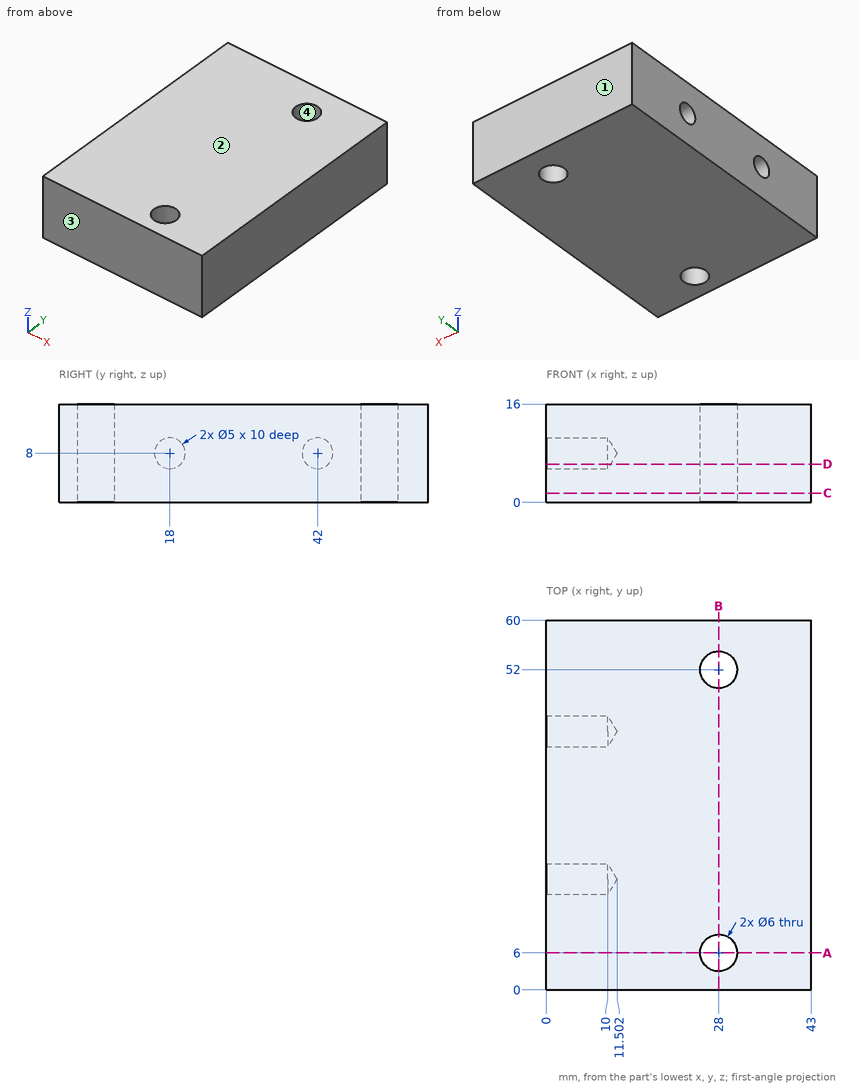
The drawing under review shows one solid part. Ordinate dimensions are in mm from its lowest x, y, z. Round coordinates to 2 decimals unless told otherwise and drop trailing zeros. Loops run counter-clockwise (first coordinate to the right, second up) from the corner with the lowest first, then second, coordinate; pieces in that order, holes last. Notation, with made-up numbers: M 27,-12.5 L 82,-12.5 A32 ccw 82,26.5 Z; hole C 83,82 d11. An arc over 180 degrees is marked long. Answer as CSV lines item,"result". Start each with the question number.
Item 1: Consider section A-A (y = 6). Write out the cut boundary in (x, z), then the cut area to 3 significant figures.
Item 2: Consider section D-D (z = 6.25). State how many separate pieces and enclosed holes the cut face has, then the cut area to 3 significant figures.
Item 3: Wall thickness on line 1 (Y direction, x = 7.75, z = 8); line 2 (Z direction, x = 6, y = 18): over which ranges is each line inside the solid? List them lowest first. Write a range as [from, to].
Item 4: Consider section B-B (x = 28). Write out the cut boundary in (y, z).
Item 5: Mouldability with a two-part tool opening along Y and no side actions: class the marked faces 1, 2, 3 and 4 as released by +Y, released by -Y, zero draft, split by the parting line, or undercut.
Item 6: Consider section C-C (z = 1.5). Write out the cut boundary in (x, y), then the cut area to 3 significant figures.
Answer:
1,outline,"M 0,0 L 25,0 L 25,16 L 0,16 Z; M 31,0 L 43,0 L 43,16 L 31,16 Z"
1,area,"592 mm^2"
2,separate pieces,"1"
2,enclosed holes,"2"
2,area,"2,450 mm^2"
3,line 1,"y = [0, 15.5], [20.5, 39.5], [44.5, 60]"
3,line 2,"z = [0, 5.5], [10.5, 16]"
4,outline,"M 0,0 L 3,0 L 3,16 L 0,16 Z; M 9,0 L 49,0 L 49,16 L 9,16 Z; M 55,0 L 60,0 L 60,16 L 55,16 Z"
5,face 1,"released by +Y"
5,face 2,"zero draft"
5,face 3,"released by -Y"
5,face 4,"undercut"
6,outline,"M 0,0 L 43,0 L 43,60 L 0,60 Z; hole C 28,6 d6; hole C 28,52 d6"
6,area,"2,520 mm^2"
